Geometry: final body of the model. Coordinates: model frame, mm. Face numbers are marked on the shaded views. A direction names the side the tool comes from. Round coordinates to 2 decimals unless told otherwise and drop trailing zeros. Order: outer loops, then holes, each group sorted by start corner. A loop starts at its lowest first (then second) coordinate and runs counter-clockwise, first axis right, second up. Notation, with made-up numbers: (58.25, 20.5) - (94.25, 20.5) arc R23 cw to (94.25, 45.5) - close; hole circle Ø8 at (35.25, 41). An arc over 180 degrees is marked (long way). Put each result on its own line as item: value. Start each with the question number.
(1) Section B-B (y = 62). Output: boundary loops of the cut face in (x, z), and give its area (3 significant figures).
(2) Access query for the marked faces 1, 2 and 3. Directions: +Z, -Z, +X, -X, +Y, -Y. A direction counts if a zero-diameter tool reaches every point of the face in a straight line with its end or side. Return the directions, or none.
(3) Section A-A (z = 3.75). Count the separate pieces of the cut face and the enclosed holes in it, and give its area (3 significant figures).
(4) Material intervals for L1, parallel to Z at x = 3, y = 6; L2, parallel to X at y = 37, z = 0.5; L3, parallel to Z at x = 6.25, y = 2.15, sorted ascending. Write a range as [from, to].
(5) Section C-C (x = 6.25). Output: boundary loops of the cut face in (y, z), and give its area (3 significant figures).
(6) Section D-D (y = 6.25). Output: boundary loops of the cut face in (x, z).
(7) Pull-direction query (Y, two-part tool) for the marked faces 4, 5, 6 and 7; classes: released by +Y, released by -Y, zero draft, split by the parting line, or undercut.
(8) Pin query (flat end, axial travel): P1, Ø12, axis at x = 20, y = 12.5, coming from the -Z side; P2, Ø2, axis at x = 16, z = 4.5, coming from the +Y side; P3, Ø4, axis at y = 35, z = 5, coming from the -X side; P4, Ø2.5, axis at y = 76.5, z = 4.5, coming from the +X side. Return the tip coordinate at first contact, or that it passes through.
from build123d import *

# Parameters (mm, degrees)
AUFSATZ_LINEAR_AUSTRAGEN1_DEPTH = 7.5
SCHNITT_LINEAR_AUSTRAGEN1_DEPTH = 10
SKIZZE7_R                       = 3
SCHNITT_LINEAR_AUSTRAGEN4_DEPTH = 84.113251049
M4_GEWINDEBOHRUNG1_D            = 3.3
M4_GEWINDEBOHRUNG1_DEPTH        = 7.5
M4_GEWINDEBOHRUNG1_TIP          = 0.991420021
SKIZZE9_OUTSIDE_W               = 26.654
SKIZZE9_OUTSIDE_H               = 99.154
SKIZZE9_OUTSIDE_R               = 1.5
SCHNITT_LINEAR_AUSTRAGEN5_DEPTH = 6
SKIZZE10_OUTSIDE_W              = 26.654
SKIZZE10_OUTSIDE_H              = 99.154
SKIZZE10_OUTSIDE_R              = 1.5
SCHNITT_LINEAR_AUSTRAGEN6_DEPTH = 6


with BuildPart() as part:
    # Skizze1 → Aufsatz-Linear austragen1 (new body)
    with BuildSketch(Plane.XY):
        with BuildLine():
            Line((-8.75, 75), (-3.25, 75))
            ThreePointArc((-3.25, 75), (-0.951902961, 74.048097039), (0, 71.75))
            Line((0, 71.75), (0, 2))
            Line((0, 2), (2, 0))
            Line((2, 0), (10.5, 0))
            Line((10.5, 0), (12.5, 2))
            Line((12.5, 2), (12.5, 71.75))
            ThreePointArc((12.5, 71.75), (13.451902961, 74.048097039), (15.75, 75))
            Line((15.75, 75), (21.25, 75))
            Line((21.25, 75), (21.25, 80))
            Line((21.25, 80), (-8.75, 80))
            Line((-8.75, 80), (-8.75, 75))
        make_face()
    extrude(amount=AUFSATZ_LINEAR_AUSTRAGEN1_DEPTH)

    # Skizze2 → Schnitt-Linear austragen1 (cut)
    with BuildSketch(Plane.XY.offset(7.5)):
        with BuildLine():
            Line((10, 71.25), (10, 13.75))
            ThreePointArc((10, 13.75), (6.25, 10), (2.5, 13.75))
            Line((2.5, 13.75), (2.5, 71.25))
            ThreePointArc((2.5, 71.25), (6.25, 75), (10, 71.25))
        make_face()
    extrude(amount=-SCHNITT_LINEAR_AUSTRAGEN1_DEPTH, mode=Mode.SUBTRACT)

    # Skizze7 → Schnitt-Linear austragen4 (cut, through all)
    with BuildSketch(Plane(origin=(12.5, 0, 0), x_dir=(0, 0, -1), z_dir=(1, 0, 0))):
        with Locations(Location((-3.75, 6.25, 0), (0, 0, 90))):
            Circle(SKIZZE7_R)
    extrude(amount=-SCHNITT_LINEAR_AUSTRAGEN4_DEPTH, mode=Mode.SUBTRACT)

    # M4 Gewindebohrung1
    with Locations(Plane(origin=(6.25, 0, 3.75), x_dir=(0, 0, -1), z_dir=(0, -1, 0))):
        with Locations((0, 0)):
            Hole(M4_GEWINDEBOHRUNG1_D / 2, depth=M4_GEWINDEBOHRUNG1_DEPTH)
            with Locations((0, 0, -(M4_GEWINDEBOHRUNG1_DEPTH + M4_GEWINDEBOHRUNG1_TIP / 2))):  # 118° drill point
                Cone(0, M4_GEWINDEBOHRUNG1_D / 2, M4_GEWINDEBOHRUNG1_TIP, mode=Mode.SUBTRACT)

    # Skizze9 outside → Schnitt-Linear austragen5 (cut)
    with BuildSketch(Plane(origin=(21.25, 0, 0), x_dir=(0, 0, -1), z_dir=(1, 0, 0))):
        with Locations((-3.75, 40)):
            Rectangle(SKIZZE9_OUTSIDE_W, SKIZZE9_OUTSIDE_H)
        with Locations((-3.75, 77.5)):
            Circle(SKIZZE9_OUTSIDE_R, mode=Mode.SUBTRACT)
    extrude(amount=-SCHNITT_LINEAR_AUSTRAGEN5_DEPTH, mode=Mode.SUBTRACT)

    # Skizze10 outside → Schnitt-Linear austragen6 (cut)
    with BuildSketch(Plane.ZY.offset(8.75)):
        with Locations((3.75, 40)):
            Rectangle(SKIZZE10_OUTSIDE_W, SKIZZE10_OUTSIDE_H)
        with Locations(Location((3.75, 77.5, 0), (0, 0, 180))):
            Circle(SKIZZE10_OUTSIDE_R, mode=Mode.SUBTRACT)
    extrude(amount=-SCHNITT_LINEAR_AUSTRAGEN6_DEPTH, mode=Mode.SUBTRACT)

    # Skizze11 → Rotation2 (revolve)
    with BuildSketch(Plane(origin=(0, 77.5, 0), x_dir=(1, 0, 0), z_dir=(0, 1, 0))):
        with BuildLine():
            Line((18.25, -2.25), (18.25, -3.75))
            Line((18.25, -3.75), (23.848076211, -3.75))
            ThreePointArc((23.848076211, -3.75), (21.624533347, -0.852222521), (18.25, -2.25))
        make_face()
        with BuildLine():
            Line((-5.75, -2.25), (-5.75, -3.75))
            Line((-5.75, -3.75), (-11.348076211, -3.75))
            ThreePointArc((-11.348076211, -3.75), (-9.124533347, -0.852222521), (-5.75, -2.25))
        make_face()
    revolve(axis=Axis((-8.75, 77.5, 3.75), (1, 0, 0)))


solid = part.part
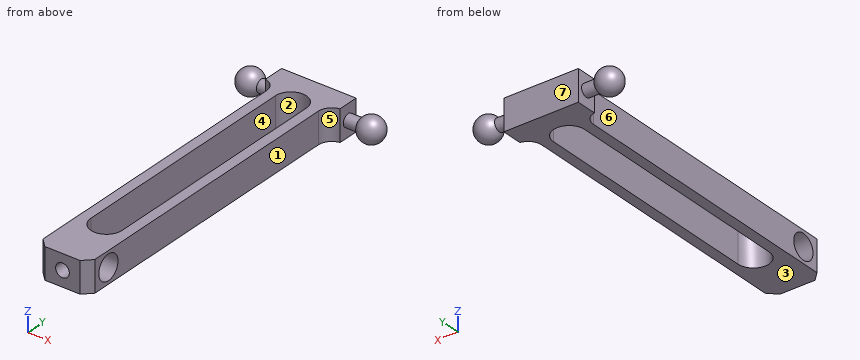
Checks:
1. outline: (0, 0) - (2.5, 0) - (2.5, 7.5) - (0, 7.5) - close; (10, 0) - (12.5, 0) - (12.5, 7.5) - (10, 7.5) - close
1. area: 37.5 mm²
2. face 1: +Z, -Z, +X, -Y
2. face 2: +Z, -Z
2. face 3: -Z, +X, -X, +Y, -Y
3. separate pieces: 3
3. enclosed holes: 1
3. area: 540 mm²
4. L1: z = [0, 0.76], [6.74, 7.5]
4. L2: x = [0, 2.5], [10, 12.5]
4. L3: z = [0, 2.1], [5.4, 7.5]
5. outline: (0, 0) - (10, 0) - (10, 7.5) - (0, 7.5) - (0, 5.4) - (3.74, 5.4) arc R3 cw (long way) to (3.74, 2.1) - (0, 2.1) - close; (75, 0) - (80, 0) - (80, 7.5) - (75, 7.5) - close
5. area: 73.0 mm²
6. outline: (0, 0) - (12.5, 0) - (12.5, 0.75) - (0, 0.75) - close; (0, 6.75) - (12.5, 6.75) - (12.5, 7.5) - (0, 7.5) - close
7. face 4: undercut
7. face 5: released by -Y
7. face 6: zero draft
7. face 7: released by +Y
8. P1: passes through
8. P2: stops at y = 80
8. P3: stops at x = 0
8. P4: stops at x = 23.85
